from build123d import *

# Parameters (mm, degrees)
CROQUIS1_W              = 40
CROQUIS1_H              = 35.6
SALIENTE_EXTRUIR1_DEPTH = 1
CROQUIS2_W              = 6.658598016
CROQUIS2_H              = 3.439056118
CROQUIS2_W_2            = 4.643913986
CROQUIS2_H_2            = 5.561026915
CROQUIS2_W_3            = 2.634170644
CROQUIS2_H_3            = 3.365884712
CROQUIS2_W_4            = 4.463455813
CROQUIS2_H_4            = 1.097571101
CROQUIS2_W_5            = 1.317085322
CROQUIS2_H_5            = 3.256127602
CROQUIS2_W_6            = 3.585398932
CROQUIS2_H_6            = 4.317112999
CROQUIS2_W_7            = 2.121970796
CROQUIS2_H_7            = 4.170770186
CROQUIS2_W_8            = 2.195142203
CROQUIS2_W_9            = 1.390256729
CROQUIS2_H_8            = 2.560999237
CROQUIS2_W_10           = 3.219541898
CROQUIS2_H_9            = 1.536599542
CROQUIS2_H_10           = 1.628063801
CROQUIS2_H_11           = 1.682942356
CROQUIS2_W_11           = 1.463428135
CROQUIS2_H_12           = 2.085385093
SALIENTE_EXTRUIR2_DEPTH = 1
CROQUIS3_W              = 4.658598016
CROQUIS3_H              = 1.439056118
SALIENTE_EXTRUIR3_DEPTH = 1


with BuildPart() as part:
    # Croquis1 → Saliente-Extruir1 (new body)
    with BuildSketch(Plane(origin=(0, 0, 0), x_dir=(1, 0, 0), z_dir=(0, 1, 0))):
        with Locations((-12.948868654, -4.565292662)):
            Rectangle(CROQUIS1_W, CROQUIS1_H)
    extrude(amount=SALIENTE_EXTRUIR1_DEPTH)

    # Croquis2 → Saliente-Extruir2 (add)
    with BuildSketch(Plane(origin=(0, 1, 0), x_dir=(1, 0, 0), z_dir=(0, 1, 0))):
        with Locations((-13.387897095, -3.650650078)):
            Rectangle(CROQUIS2_W, CROQUIS2_H)
        with Locations((-2.321956993, -14.736118204)):
            Rectangle(CROQUIS2_W_2, CROQUIS2_H_2)
        with Locations((-23.375794119, -13.638547102)):
            Rectangle(CROQUIS2_W_3, CROQUIS2_H_3)
        with Locations((-23.412379823, -10.089733874)):
            Rectangle(CROQUIS2_W_4, CROQUIS2_H_4)
        with Locations((-19.717223781, -8.461670073)):
            Rectangle(CROQUIS2_W_5, CROQUIS2_H_5)
        with Locations((-17.924524315, -17.480045957)):
            Rectangle(CROQUIS2_W_6, CROQUIS2_H_6)
        with Locations((-20.119666518, 5.715289989)):
            Rectangle(CROQUIS2_W_7, CROQUIS2_H_7)
        with Locations((-8.961026986, 5.715289989)):
            Rectangle(CROQUIS2_W_8, CROQUIS2_H_7)
        with Locations((2.490298175, -19.382502534)):
            Rectangle(CROQUIS2_W_9, CROQUIS2_H_8)
        with Locations((-2.302428969, -9.870219653)):
            Rectangle(CROQUIS2_W_10, CROQUIS2_H_9)
        with Locations((-2.302428969, -7.647638173)):
            Rectangle(CROQUIS2_W_10, CROQUIS2_H_10)
        with Locations((-2.302428969, -5.260421027)):
            Rectangle(CROQUIS2_W_10, CROQUIS2_H_11)
        with Locations((-10.790312155, -10.9129122)):
            Rectangle(CROQUIS2_W_11, CROQUIS2_H_12)
    extrude(amount=SALIENTE_EXTRUIR2_DEPTH)

    # Croquis3 → Saliente-Extruir3 (add)
    with BuildSketch(Plane(origin=(0, 2, 0), x_dir=(1, 0, 0), z_dir=(0, 1, 0))):
        with Locations((-13.387897095, -3.650650078)):
            Rectangle(CROQUIS3_W, CROQUIS3_H)
    extrude(amount=SALIENTE_EXTRUIR3_DEPTH)


solid = part.part
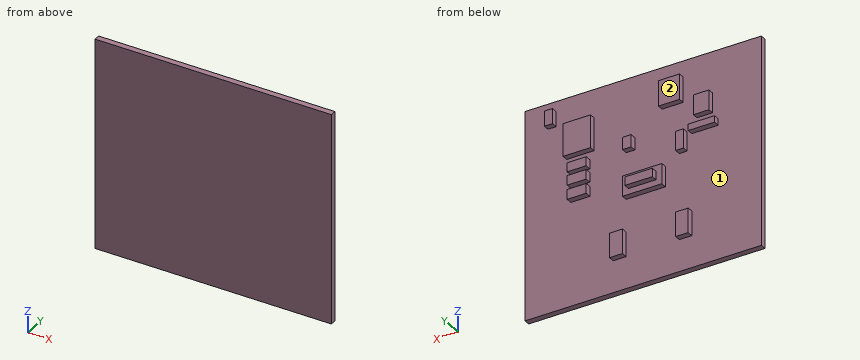
Check sheet for the modelled part. Datum: model origin and axes. Units: mm. Face numbers are marked on the shaded views. Give positions to 0.01 mm unless a question says otherwise; leave off trailing zeros. Loops run counter-clockwise (first coordinate to the right, second up) from the corner with the lowest first, then second, coordinate; pieces in that order, holes last. Notation, with made-up numbers: M -17.5,-7.5 L 13.5,-7.5 A13 cw 13.5,-0.5 Z; hole C 8.25,-21 d1. An arc over 180 degrees is marked long. Use a Markdown table: item, result. Add a question column.
Q1. Mould release check, pull along X, two halves, no side actions. Record for the marked faces 1 and 2: pulls with the +X half, pulls with the -X half, needs draft (parallel to the pull), parting line crosses it, or undercut.
Q2. Go/stop test with flat-tipped pins: pin 1 (1.1 mm diameter, centred on y = 2.5, z = 4, fed in from -X); pin 2 (0.5 mm diameter, centred on y = 1.5, z = 15.5, fed in from -X); pin 3 (0.8 mm diameter, centred on x = -22.5, y = 1.5, fed in from +Z). Record where each tip stops, or that it passes through.
Q3. Sectioned sample at C-C, the plane z = -2.5. Record the cut outline in (x, y).
Q4. Sectioned sample at B-B, the plane y = 1.45. Give the number of separate pieces and of enclosed holes in the cut face, then the cut area to 3 significant figures.
Q5. Sectioned sample at A-A, the plane x = -22.5. Record the cut outline in (y, z).
Q6. Scan lines: line 1 along Z through (x, y) = (-2, 1.4); line 2 along X through (y, z) = (1.15, 19.5); line 3 along X through (y, z) = (1.05, 9.5). Record each from-to range of solid material in increasing order. Write a range as [from, to].
Q7. Sectioned sample at D-D, the plane x = -12. Record the cut outline in (y, z), then the cut area to 3 significant figures.
Verdict:
| question | item | result |
|---|---|---|
| 1 | face 1 | undercut |
| 1 | face 2 | needs draft |
| 2 | pin 1 | x = -16.72 |
| 2 | pin 2 | x = -24.69 |
| 2 | pin 3 | z = 15.32 |
| 3 | outline | M -32.95,0 L 7.05,0 L 7.05,1 L -32.95,1 Z |
| 4 | separate pieces | 13 |
| 4 | enclosed holes | 0 |
| 4 | area | 122 mm^2 |
| 5 | outline | M 0,-13.23 L 1,-13.23 L 1,9.54 L 2,9.54 L 2,10.64 L 1,10.64 L 1,11.96 L 2,11.96 L 2,15.32 L 1,15.32 L 1,22.37 L 0,22.37 Z |
| 6 | line 1 | [4.42, 6.1], [6.83, 8.46], [9.1, 10.64], [11.96, 17.52] |
| 6 | line 2 | [-19.72, -16.13], [1.8, 3.19] |
| 6 | line 3 | [-20.38, -19.06], [-3.91, -0.69] |
| 7 | outline | M 0,-13.23 L 1,-13.23 L 1,1.93 L 2,1.93 L 2,2.93 L 3,2.93 L 3,4.37 L 2,4.37 L 2,5.37 L 1,5.37 L 1,22.37 L 0,22.37 Z |
| 7 | area | 40.5 mm^2 |
